Could you check a few things on this model? Use its own coordinates, in mm. A direction names the side the tool comes from. Give positions to 0.01 mm unless a question says otherwise; leave off trailing zeros. Write each loop counter-clockwise with the first axis right and the second up, starting at its lowest first coordinate (ties: lowest second). Pieces come first, ordered by that corner, then holes. Notation, with made-up numbers: (43.5, 1.5) -> (93.5, 1.5) arc R25 ccw to (93.5, 28.5) -> close; hole circle Ø1 at (34, 14). An arc over 180 degrees is marked (long way). Write item = value, one per line. Start each with the question number.
```python
from build123d import *

# Parameters (mm, degrees)
BOSS_EXTRUDE1_DEPTH              = 5
SKETCH4_R                        = 2.75
POT_HOLE_DEPTH                   = 82.062316455
POT_START                        = 5
POT_INSERT_DEPTH                 = 2.5
MIDDLE_START                     = 3.5
MIDDLE_FLEXION_DEPTH             = 2.5
MIDDLE_START_2                   = 0.5
MIDDLE_EXTENSION_DEPTH           = 5.5
PROXIMAL_START                   = 0.5
PROXIMAL_FLEXION_EXTENSION_DEPTH = 5.5
SKETCH9_R                        = 0.8
SCREW_HOLES_DEPTH                = 82.062316455
CUT_EXTRUDE4_START               = 0.5
CUT_EXTRUDE4_DEPTH               = 5.5
CUT_EXTRUDE5_START               = 5
CUT_EXTRUDE5_DEPTH               = 2.5


with BuildPart() as part:
    # Sketch1 → Boss-Extrude1 (new body)
    with BuildSketch(Plane.XY):
        with BuildLine():
            Line((72.287602711, 8), (41.287602711, 8))
            Line((41.287602711, 8), (41.287602711, 10))
            Line((41.287602711, 10), (37.287602711, 10))
            Line((37.287602711, 10), (37.287602711, -10))
            Line((37.287602711, -10), (41.287602711, -10))
            Line((41.287602711, -10), (41.287602711, -8))
            Line((41.287602711, -8), (72.287602711, -8))
            ThreePointArc((72.287602711, -8), (80.287602711, 0), (72.287602711, 8))
        make_face()
    extrude(amount=BOSS_EXTRUDE1_DEPTH)

    # Sketch4 → Pot Hole (cut, through all)
    with BuildSketch(Plane.XY):
        with Locations((72.287602711, 0)):
            Circle(SKETCH4_R)
    extrude(amount=POT_HOLE_DEPTH, mode=Mode.SUBTRACT)

    # Sketch3 → Pot Insert (cut)
    with BuildSketch(Plane(origin=(28.28760271, 0, 0), x_dir=(1, 0, 0), z_dir=(0, 0, 1)).offset(POT_START)):
        Polygon((51.000000001, 0), (51.000000001, 1.5), (49.500000001, 1.5), (48.000000001, 4.5), (48.000000001, 5.5), (44.000000001, 5.5), (39.750000001, 5.5), (39.750000001, 4.5), (34.500000001, 4.5), (34.500000001, 0), (34.500000001, -4.5), (39.750000001, -4.5), (39.750000001, -5.5), (44.000000001, -5.5), (48.000000001, -5.5), (48.000000001, -4.5), (49.500000001, -1.5), (51.000000001, -1.5), align=None)
    extrude(amount=-POT_INSERT_DEPTH, mode=Mode.SUBTRACT)

    # Sketch16 → Middle Flexion (cut)
    with BuildSketch(Plane.XY.offset(MIDDLE_START)):
        with BuildLine():
            Line((65.431633901, -8), (72.287602711, -8))
            ThreePointArc((72.287602711, -8), (70.883144469, -7.875753744), (69.522310897, -7.506874262))
            Line((69.522310897, -7.506874262), (57.287602711, -3))
            Line((57.287602711, -3), (37.287602711, -3))
            Line((37.287602711, -3), (37.287602711, -5))
            Line((37.287602711, -5), (57.287602711, -5))
            Line((57.287602711, -5), (65.431633901, -8))
        make_face()
    extrude(amount=MIDDLE_FLEXION_DEPTH, mode=Mode.SUBTRACT)

    # Sketch11 → Middle Extension (cut)
    with BuildSketch(Plane.XY.offset(MIDDLE_START_2)):
        with BuildLine():
            Line((57.287602711, 5.000000001), (37.287602711, 5.000000001))
            Line((37.287602711, 5.000000001), (37.287602711, 3.000000001))
            Line((37.287602711, 3.000000001), (57.287602711, 3.000000001))
            Line((57.287602711, 3.000000001), (69.522310897, 7.506874262))
            ThreePointArc((69.522310897, 7.506874262), (70.88314447, 7.875753745), (72.287602711, 8))
            Line((72.287602711, 8), (65.4316339, 8))
            Line((65.4316339, 8), (57.287602711, 5.000000001))
        make_face()
    extrude(amount=MIDDLE_EXTENSION_DEPTH, mode=Mode.SUBTRACT)

    # Sketch8 → Proximal Flexion/Extension (cut)
    with BuildSketch(Plane.XY.offset(PROXIMAL_START)):
        with BuildLine():
            ThreePointArc((47.287602711, 2), (49.287602711, 0), (47.287602711, -2))
            Line((47.287602711, -2), (37.287602711, -2))
            Line((37.287602711, -2), (37.287602711, 0))
            Line((37.287602711, 0), (37.287602711, 2))
            Line((37.287602711, 2), (47.287602711, 2))
        make_face()
    extrude(amount=PROXIMAL_FLEXION_EXTENSION_DEPTH, mode=Mode.SUBTRACT)

    # Sketch9 → Screw Holes (cut, through all)
    with BuildSketch(Plane.XY):
        with Locations((47.287602711, 0)):
            Circle(SKETCH9_R)
        with Locations((56.787602711, -6.25)):
            Circle(SKETCH9_R)
        with Locations((39.287602711, -6.25)):
            Circle(SKETCH9_R)
        with Locations((55.287602711, 0)):
            Circle(SKETCH9_R)
        with Locations((39.287602711, 6.25)):
            Circle(SKETCH9_R)
        with Locations((56.787602711, 6.25)):
            Circle(SKETCH9_R)
    extrude(amount=SCREW_HOLES_DEPTH, mode=Mode.SUBTRACT)

    # Sketch12 → Cut-Extrude4 (cut)
    with BuildSketch(Plane.XY.offset(CUT_EXTRUDE4_START)):
        with BuildLine():
            Line((62.787602711, 2), (60.787602711, 2))
            Line((60.787602711, 2), (55.287602711, 2))
            ThreePointArc((55.287602711, 2), (53.287602711, 0), (55.287602711, -2))
            Line((55.287602711, -2), (60.787602711, -2))
            Line((60.787602711, -2), (60.787602711, -6.289287793))
            Line((60.787602711, -6.289287793), (65.431633901, -8))
            Line((65.431633901, -8), (72.287602711, -8))
            ThreePointArc((72.287602711, -8), (70.883144469, -7.875753745), (69.522310897, -7.506874262))
            Line((69.522310897, -7.506874262), (62.787602711, -5.026023675))
            Line((62.787602711, -5.026023675), (62.787602711, 2))
        make_face()
    extrude(amount=CUT_EXTRUDE4_DEPTH, mode=Mode.SUBTRACT)

    # Sketch13 → Cut-Extrude5 (cut)
    with BuildSketch(Plane.XY.offset(CUT_EXTRUDE5_START)):
        Polygon((62.787602711, 2), (60.787602711, 2), (60.787602711, 4.289287794), (62.787602711, 5.026023675), align=None)
    extrude(amount=-CUT_EXTRUDE5_DEPTH, mode=Mode.SUBTRACT)


solid = part.part
```
(1) I'm going to push flat-ended pins straight in: pin 1 (1.1 mm diameter, centred on y = 5, z = 4, fed in from +X); pin 2 (1.5 mm diameter, centred on x = 46, z = 1, fed in from +Y); pin 3 (3 mm diameter, centred on x = 72.5, z = 4, fed in from -Y); pin 4 (3.5 mm diameter, centred on x = 72.29, y = 0, fed in from -Z). Where does each tip first touch, or does it pass through?
(2) We'd pull the mould along Y, two halves only. Please class faces 4 (the flat face through (54, 8, 2)), 5 (the flat face through (39, -10, 2)), 6 (the flat face through (65, -4.5, 4)): released by +Y, released by -Y, zero draft, split by the parting line, or undercut.
(3) Imagine slicing it at A-A (z = 1). State how many separate pieces and enclosed holes the cut face has, then the cut area to 3 significant figures.
(4) Imagine slicing it at B-B (y = 0). Please give me the cut outline in (x, z), then the cut area to 4 significant figures.
(5) If I drill on line 1 along Y through (x, z) = (47, 3.65); line 2 along X through (y, z) = (0, 1.35); line 3 along Y through (x, z) = (55, 2.05), over which ranges is the centre line in solid material (lowest first)? Write a range as from..to.
(6) On a 3-axis mill with a long thin cutter (end or side, diameter ignored), from which of +Z, -Z, +X, -X, +Y, -Y can I reach the whole of each face in a straight line? I mean faces 1 (the flat face through (53, -8, 2)), 2 (the flat face through (68.038, 5, 4)), 3 (the flat face through (47, -3, 4)). Say none if no direction works.
(7) Imagine slicing it at C-C (x = 42.5). Please give me the cut outline in (y, z), then the cut area to 3 significant figures.
Answers below:
q1.pin_1 = 78.94
q1.pin_2 = 8
q1.pin_3 = -8
q1.pin_4 = through
q2.face_4 = released by +Y
q2.face_5 = released by -Y
q2.face_6 = undercut
q3.separate_pieces = 2
q3.enclosed_holes = 5
q3.area = 480 mm^2
q4.outline = (37.29, 0) -> (46.49, 0) -> (46.49, 0.5) -> (37.29, 0.5) -> close; (48.09, 0) -> (54.49, 0) -> (54.49, 0.5) -> (53.29, 0.5) -> (53.29, 5) -> (49.29, 5) -> (49.29, 0.5) -> (48.09, 0.5) -> close; (56.09, 0) -> (69.54, 0) -> (69.54, 2.5) -> (62.79, 2.5) -> (62.79, 0.5) -> (56.09, 0.5) -> close; (75.04, 0) -> (80.29, 0) -> (80.29, 5) -> (79.29, 5) -> (79.29, 2.5) -> (75.04, 2.5) -> close
q4.area = 61.65 mm^2
q5.line_1 = -8..-5, -3..-2, 2..3, 5..8
q5.line_2 = 49.29..53.29, 62.79..69.54, 75.04..80.29
q5.line_3 = -8..-1.98, 1.98..3, 5..8
q6.face_1 = +Z, -Z, +X, -Y
q6.face_2 = +Z
q6.face_3 = +Z, -X
q7.outline = (-8, 0) -> (8, 0) -> (8, 5) -> (5, 5) -> (5, 0.5) -> (3, 0.5) -> (3, 5) -> (2, 5) -> (2, 0.5) -> (-2, 0.5) -> (-2, 5) -> (-3, 5) -> (-3, 3.5) -> (-5, 3.5) -> (-5, 5) -> (-8, 5) -> close
q7.area = 50.0 mm^2
